Could you check a few things on this model? Use its own coordinates, in mm. Face numbers are marked on the shaded views. Coordinates: 2 decimals unless noted, no trailing zeros. Write each loop counter-clockwise with the first axis right and the second up, starting at its lowest first coordinate (ties: lowest second). Pieces come first, ordered by that corner, then holes.
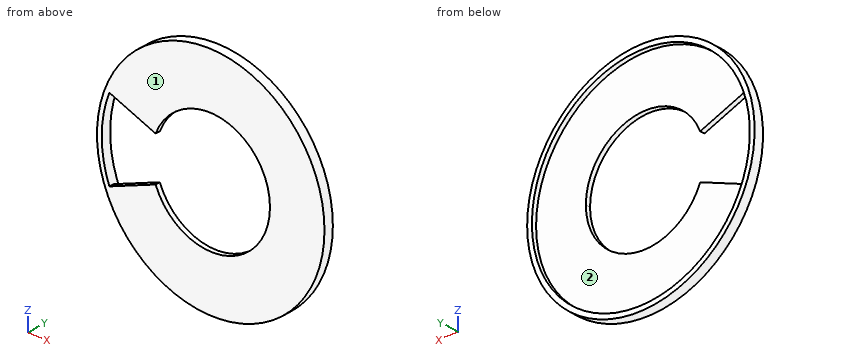
```python
from build123d import *

# Parameters (mm, degrees)
SKETCH1_R           = 48
SKETCH1_R_2         = 46
BOSS_EXTRUDE1_DEPTH = 4
BOSS_EXTRUDE2_DEPTH = 2


with BuildPart() as part:
    # Sketch1 → Boss-Extrude1 (new body)
    with BuildSketch(Plane(origin=(0, 0, 0), x_dir=(1, 0, 0), z_dir=(0, 1, 0))):
        Circle(SKETCH1_R)
        Circle(SKETCH1_R_2, mode=Mode.SUBTRACT)
    extrude(amount=BOSS_EXTRUDE1_DEPTH)

    # Sketch1_3 → Boss-Extrude2 (add)
    with BuildSketch(Plane(origin=(0, 0, 0), x_dir=(1, 0, 0), z_dir=(0, 1, 0))):
        with BuildLine():
            ThreePointArc((25, 0), (4.6631009, -24.561259943), (-23.2604392, -9.162530668))
            Line((-23.2604392, -9.162530668), (-42.799208127, -16.859056429))
            ThreePointArc((-42.799208127, -16.859056429), (8.580105656, -45.192718295), (46, 0))
            ThreePointArc((46, 0), (8.580105656, 45.192718295), (-42.799208127, 16.859056429))
            Line((-42.799208127, 16.859056429), (-23.2604392, 9.162530668))
            ThreePointArc((-23.2604392, 9.162530668), (4.6631009, 24.561259943), (25, 0))
        make_face()
    extrude(amount=BOSS_EXTRUDE2_DEPTH)


solid = part.part
```
Item 1: I want a section at C-C, the plane z = 28. List the corners of the cut face in (x, y) for me.
Item 2: I want a section at D-D, the plane x = -33. List the corners of the cut face in (y, z) for me.
Item 3: If we mould it in two halves opening along Z, with no side actions, what happens to the marked faces 1 and 2? For each: released by +Z, released by -Z, zero draft, split by the parting line, or undercut.
Item 4: Will this pin go through, and if not, where does the flat tip stop? pin 1 Ø2 at (y, z) = (3.5, -37) entering from -X.
Item 5: If I drill on line 1 along X through (y, z) = (3.05, 0); line 2 along X through (y, z) = (1.75, 0), over which ranges is the centre line in solid material (lowest first)?
Item 6: I want a section at B-B, the plane y = 1.1. List the corners of the cut face in (x, z) for me.
Item 7: I want a section at A-A, the plane x = 0. List the corners of the cut face in (y, z) for me, then the cut area to 3 significant figures.
Taken from the geometry:
1. outline: (-38.99, 0) - (38.99, 0) - (38.99, 4) - (36.5, 4) - (36.5, 2) - (-36.5, 2) - (-36.5, 4) - (-38.99, 4) - close
2. outline: (0, -34.86) - (4, -34.86) - (4, -32.05) - (2, -32.05) - (2, -13) - (0, -13) - close; (0, 13) - (2, 13) - (2, 32.05) - (4, 32.05) - (4, 34.86) - (0, 34.86) - close
3. face 1: zero draft
3. face 2: undercut
4. pin 1: stops at x = -31.75
5. line 1: x = -48 to -46, 46 to 48
5. line 2: x = -48 to -46, 25 to 48
6. outline: circle Ø96 at (0, 0); hole (-42.8, -16.86) - (-23.26, -9.16) arc R25 ccw (long way) to (-23.26, 9.16) - (-42.8, 16.86) arc R46 ccw to start
7. outline: (0, -48) - (4, -48) - (4, -46) - (2, -46) - (2, -25) - (0, -25) - close; (0, 25) - (2, 25) - (2, 46) - (4, 46) - (4, 48) - (0, 48) - close
7. area: 100 mm2
